Read the model definition and answer for the solid it produces. Units are mm, in the model's axes. A direction names the side the tool comes from. Give positions to 0.01 mm unless a question says otherwise; leave off trailing zeros. Order: outer loops, then holes, each group sorted by start corner. A loop starts at its lowest first (then second) coordinate and runs counter-clockwise, first axis right, second up. Notation, with made-up numbers: M 77.5,26 L 114.5,26 A7 cw 114.5,35 Z; hole C 22,47 d4. An arc over 180 degrees is marked long. One line per item, written item: value. Start each with the question number.
Autodesk Inventor part; units mm, degrees
ref_plane "YZ Plane" through (0, 0, 0) normal (1, 0, 0) x (0, 1, 0)
ref_plane "XZ Plane" through (0, 0, 0) normal (0, 1, 0) x (-1, 0, 0)
ref_plane "XY Plane" through (0, 0, 0) normal (0, 0, 1) x (1, 0, 0)
sketch "Эскиз1" plane through (0, 0, 0) normal (0, 1, 0) x (-1, 0, 0)
  line L0 (150, 150) -> (-150, 150)
  line L1 (-150, 150) -> (-150, -150)
  line L2 (-150, -150) -> (150, -150)
  line L3 (150, -150) -> (150, 150)
  circle A0 centre (0, 0) radius 150
  line L4 (-106, -106) -> (105.4385, -106)
  line L5 (105.4385, -106) -> (105.4385, 106.6899)
  line L6 (105.4385, 106.6899) -> (-106, 106.6899)
  line L7 (-106, 106.6899) -> (-106, -106)
  line L8 (82, 90) -> (-80, 90)
  line L9 (-95, 75) -> (-95, -75)
  line L10 (-80, -90) -> (82, -90)
  line L11 (95, -77) -> (95, 77)
  arc A1 (95, 77) -> (82, 90) centre (82, 77) ccw
  arc A2 (82, -90) -> (95, -77) centre (82, -77) ccw
  line L12 (72, 84.5) -> (12, 84.5)
  line L13 (12, 69.5) -> (72, 69.5)
  line L14 (-80, 90) -> (-82, 90)
  line L15 (-95, 77) -> (-95, 75)
  arc A3 (-82, 90) -> (-95, 77) centre (-82, 77) ccw
  line L16 (-80, -90) -> (-82, -90)
  line L17 (-95, -77) -> (-95, -75)
  arc A4 (-95, -77) -> (-82, -90) centre (-82, -77) ccw
  line L18 (76.9408, 68) -> (82, 68)
  line L19 (82, 68) -> (-82, 68)
  line L20 (-82, 86) -> (82, 86)
  line L21 (82, -68) -> (-82, -68)
  line L22 (-82, -68) -> (-82, -86)
  line L23 (-82, -86) -> (82, -86)
  line L24 (-82, 68) -> (-72, 68)
  line L25 (-72, 86) -> (-82, 86)
  line L26 (-82, 86) -> (-82, 68)
  line L27 (-82, -86) -> (-72, -86)
  line L28 (-72, -68) -> (-82, -68)
  line L29 (-82, -68) -> (-82, -86)
  line L30 (82, -86) -> (72, -86)
  line L31 (72, -68) -> (82, -68)
  line L32 (82, -68) -> (82, -86)
  line L33 (72, 68) -> (82, 68)
  line L34 (82, 68) -> (82, 86)
  line L35 (82, 86) -> (72, 86)
  line L36 (42, 68) -> (54.5, 68)
  line L37 (42, 8) -> (17, 8)
  line L38 (29.5, 8) -> (29.5, 68)
  line L39 (29.5, 68) -> (54.5, 68)
  line L40 (54.5, 68) -> (54.5, 8)
  line L41 (42, -8) -> (17, -8)
  line L42 (29.5, -8) -> (29.5, -68)
  line L43 (29.5, -68) -> (54.5, -68)
  line L44 (54.5, -68) -> (54.5, -8)
  line L45 (-42, 68) -> (-29.5, 68)
  line L46 (-54.5, 8) -> (-54.5, 68)
  line L47 (-54.5, 68) -> (-29.5, 68)
  line L48 (-29.5, 68) -> (-29.5, 8)
  line L49 (-54.5, -8) -> (-54.5, -68)
  line L50 (-54.5, -68) -> (-29.5, -68)
  line L51 (-29.5, -68) -> (-29.5, -8)
  line L52 (75.5, -84.5) -> (8.5, -84.5)
  line L53 (8.5, -84.5) -> (8.5, -69.5)
  line L54 (8.5, -69.5) -> (75.5, -69.5)
  line L55 (75.5, -69.5) -> (75.5, -84.5)
  line L56 (0, -86) -> (0, -44.6693) construction
  line L57 (-75.5, -84.5) -> (-8.5, -84.5)
  line L58 (-8.5, -84.5) -> (-8.5, -69.5)
  line L59 (-8.5, -69.5) -> (-75.5, -69.5)
  line L60 (-75.5, -69.5) -> (-75.5, -84.5)
  line L61 (75.5, 84.5) -> (8.5, 84.5)
  line L62 (8.5, 84.5) -> (8.5, 69.5)
  line L63 (8.5, 69.5) -> (75.5, 69.5)
  line L64 (75.5, 69.5) -> (75.5, 84.5)
  line L65 (-8.5, 84.5) -> (-8.5, 69.5)
  line L66 (-8.5, 69.5) -> (-75.5, 69.5)
  line L67 (-75.5, 69.5) -> (-75.5, 84.5)
  line L68 (-75.5, 84.5) -> (-8.5, 84.5)
  line L69 (54.5, 8) -> (29.5, 8)
  line L70 (17, 8) -> (17, -8)
  line L71 (29.5, -8) -> (54.5, -8)
  line L72 (42, -8) -> (42, 8)
  line L73 (-54.5, 8) -> (-54.5, -8)
  line L74 (-29.5, -8) -> (-29.5, 8)
  line L75 (20, -40) -> (-20, -40)
  line L76 (-20, -40) -> (-20, 40)
  line L77 (-20, 40) -> (20, 40)
  line L78 (20, 40) -> (20, -40)
  line L79 (20, 25) -> (20, 40)
  line L80 (20, 30) -> (20, 40)
  line L81 (-10, -10) -> (10, -10)
  line L82 (10, -10) -> (10, 10)
  line L83 (10, 10) -> (-10, 10)
  line L84 (-10, 10) -> (-10, -10)
  point P0 (-95, -90)
  point P1 (-95, 90)
  point P2 (95, -90)
  point P3 (-12, -77)
  point P4 (12, -77)
  point P5 (12, 77)
  point P6 (72, 77)
  point P7 (42, 8)
  point P8 (42, -8)
  point P9 (-42, -69.5)
  point P10 (42, -8)
  point P11 (-9, 0)
  point P12 (42, 0)
  point P13 (29.5, 0)
  point P14 (-42, -69.5)
  point P15 (42, -69.5)
  dimension "d2" = 300
  dimension "d3" = 300
  dimension "d8" = 190
  dimension "d9" = 180
  dimension "d10" = 13
  dimension "d11" = 13
  dimension "d31" = 13
  dimension "d32" = 13
  dimension "d41" = 15
  dimension "d42" = 24
  dimension "d47" = 25
  dimension "d51" = 25
  dimension "d52" = 16
  dimension "d112" = 67
  dimension "d123" = 40
  dimension "d124" = 80
  dimension "d147" = 20
  dimension "d148" = 20
  dimension "d156" = 84
extrude "Выдавливание1" add sketch "Эскиз1" along normal blind 4 contours A1 L11 A2 L10 L16 A4 L17 L9 L15 A3 L14 L8 | L40 L69 L37 L38 L19 | L38 L37 L78 L77 L76 L75 L41 L42 L21 L51 L74 L48 L19 | L72 L41 L78 L37 | L48 L74 L51 L21 L49 L73 L46 L19 | L71 L44 L21 L42 L41 | L78 L41 L70 L37 | L37 L70 L41 L78 L75 L76 L77 | L84 L83 L82 L81
sketch "Эскиз2" plane through (0, 0, 0) normal (0, -1, 0) x (1, 0, 0)
  line L0 (-82, -68) -> (-82, -86)
  line L1 (-95, -77) -> (-95, 77)
  line L2 (-95, -68) -> (-95, -56.3368)
  line L3 (-95, -45) -> (-95, -68) construction
  line L4 (-95, -68) -> (-80, -68) construction
  line L5 (-95, -63) -> (-95, -68)
  line L6 (-95, -50) -> (-95, -45)
  circle A0 centre (-80, -63) radius 1.5
  circle A1 centre (-80, -50) radius 1.5
  line L7 (95, 77) -> (95, -77)
  line L8 (95, -68) -> (95, -45)
  line L9 (-95, -45) -> (-95, -68)
  line L10 (82, -90) -> (-82, -90)
  circle A2 centre (80, -63) radius 1.5
  circle A3 centre (80, -50) radius 1.5
  line L11 (-95, -68) -> (-95, -63)
  line L12 (95, -63) -> (95, -68)
  line L13 (95, -45) -> (95, -50)
  line L14 (-95, -50) -> (-95, -45)
  circle A4 centre (0, -50) radius 1.5
  circle A5 centre (0, -63) radius 1.5
  line L15 (-95, 0) -> (95, 0)
  circle A6 centre (-80, 63) radius 1.5
  circle A7 centre (-80, 50) radius 1.5
  circle A8 centre (80, 63) radius 1.5
  circle A9 centre (80, 50) radius 1.5
  circle A10 centre (0, 50) radius 1.5
  circle A11 centre (0, 63) radius 1.5
  line L16 (-95, -68) -> (95, -68)
  line L17 (95, -68) -> (95, -45)
  line L18 (95, -45) -> (-95, -45)
  line L19 (-95, -45) -> (-95, -68)
  line L20 (-82, 68) -> (-95, 68)
  line L21 (-95, 68) -> (95, 68)
  line L22 (95, 68) -> (95, 45)
  line L23 (95, 45) -> (-95, 45)
  line L24 (-95, 45) -> (-95, 68)
  point P0 (0, 0)
  dimension "d64" = 23
extrude "Выдавливание2" cut sketch "Эскиз2" against normal blind 4 contours A0 | A1 | A2 | A3 | A4 | A5 | A6 | A7 | A8 | A9 | A10 | A11
sketch "Эскиз3" plane through (0, 0, 0) normal (0, -1, 0) x (1, 0, 0)
  line L0 (-95, -77) -> (-95, 77)
  line L1 (-95, 10) -> (-95, 0)
  circle A0 centre (-73, 0) radius 1.5
  circle A1 centre (-60, -13) radius 1.5
  circle A2 centre (-60, 13) radius 1.5
  line L2 (-70, -10) -> (-80, -10)
  line L3 (-60, -10) -> (-80, -10)
  line L4 (-50, -10) -> (-68, -10)
  line L5 (-70, -8) -> (-70, 8)
  line L6 (-68, 10) -> (-50, 10)
  line L7 (-50, 10) -> (-50, -10)
  arc A3 (-70, -8) -> (-68, -10) centre (-68, -8) ccw
  arc A4 (-68, 10) -> (-70, 8) centre (-68, 8) ccw
  line L8 (0, 0) -> (-42, 0)
  line L9 (-42, 0) -> (-42, 8)
  line L10 (-42, 8) -> (0, 8)
  line L11 (0, 8) -> (0, 0)
  point P0 (-70, -13)
  point P1 (-78, -10)
  point P2 (-70, 0)
  point P3 (-60, 0)
  dimension "d79" = 3
  dimension "d87" = 2
  dimension "d149" = 42
extrude "Выдавливание3" cut sketch "Эскиз3" against normal blind 4 contours A0 | A1 | A2
extrude "Выдавливание4" cut sketch "Эскиз3" against normal blind 4 contours L3 A3 L5 A4 L6 L7 L4
sketch "Эскиз4" plane through (0, 0, 0) normal (0, -1, 0) x (1, 0, 0)
  circle A0 centre (-80, 63) radius 1.5
  circle A1 centre (-78, 57.5) radius 1.5
  circle A2 centre (0, 63) radius 1.5
  circle A3 centre (-2.2, 57.5) radius 1.5
  line L0 (-47.745, 0) -> (17.0058, 0) construction
  circle A4 centre (-78, -57.5) radius 1.5
  circle A5 centre (-2.2, -57.5) radius 1.5
  point P0 (0, 0)
  dimension "d92" = 3
  dimension "d95" = 3
extrude "Выдавливание5" cut sketch "Эскиз4" against normal blind 4 contours A1 | A3 | A4 | A5
sketch "Эскиз5" plane through (0, 0, 0) normal (0, -1, 0) x (1, 0, 0)
  line L0 (82, -68) -> (-82, -68)
  line L1 (-82, -86) -> (82, -86)
  line L2 (-90.0897, 0) -> (-46.8311, 0) construction
  line L3 (0, -13.4429) -> (0, 16.6684) construction
  circle A0 centre (-87, -8.1) radius 1.5
  line L4 (-82, 68) -> (82, 68) construction
  line L5 (0, 68) -> (-4.5, 68) construction
  line L6 (-4.5, 63) -> (0, 63) construction
  line L7 (0, 63) -> (0, 68) construction
  line L8 (-17.2785, 0) -> (16.6341, 0) construction
  circle A1 centre (-8.1, 63) radius 1.5
  circle A2 centre (-87, 8.1) radius 1.5
  circle A3 centre (87, -8.1) radius 1.5
  circle A4 centre (87, 8.1) radius 1.5
  circle A5 centre (8.1, 63) radius 1.5
  circle A6 centre (-8.1, -63) radius 1.5
  circle A7 centre (8.1, -63) radius 1.5
  point P0 (0, 0)
  point P1 (-87, 0)
  dimension "d115" = 3
extrude "Выдавливание6" cut sketch "Эскиз5" against normal blind 4 contours A0
extrude "Выдавливание7" cut sketch "Эскиз5" against normal blind 4 contours A1
extrude "Выдавливание8" cut sketch "Эскиз1" along normal blind 4 contours L72 L41 L78 L37 | L78 L41 L70 L37
extrude "Выдавливание9" cut sketch "Эскиз1" along normal blind 4 contours L84 L83 L82 L81
sketch "Эскиз6" plane through (0, 4, 0) normal (0, 1, 0) x (1, 0, 0)
  line L0 (15, -37.5) -> (75, -37.5)
  line L1 (75, -37.5) -> (75, 37.5)
  line L2 (75, 37.5) -> (15, 37.5)
  line L3 (15, 37.5) -> (15, -37.5)
  line L4 (15, -37.5) -> (25, -37.5)
  line L5 (45, -37.5) -> (45, 37.5) construction
  circle A0 centre (25, 0) radius 1.5
  circle A1 centre (65, 0) radius 1.5
  point P0 (0, 0)
  dimension "d139" = 60
  dimension "d140" = 75
  dimension "d141" = 10
  dimension "d142" = 3
extrude "Выдавливание10" cut sketch "Эскиз6" against normal blind 4 contours A0 | A1
extrude "Выдавливание11" cut sketch "Эскиз5" against normal blind 10 contours A2
extrude "Выдавливание12" cut sketch "Эскиз5" against normal blind 10 contours A3 | A4 | A5 | A6 | A7
properties part number "основа"
Q1. Find section A-A, the plane x = 57. Give the vertices of the cut face in (y, z), then the cut area to 3 significant figures.
Q2. Find section B-B, the plane y = 1.6. State how many separate pieces and enclosed holes the cut face has, then the cut area to 3 significant figures.
Q3. Each of these flat-tipped pins is pushed along its axis until it touches: pin 1 (4 mm diameter, centred on x = 8.1, z = 63, fed in from -Y); pin 2 (2.5 mm diameter, centred on x = 65, z = 0, fed in from -Y); pin 3 (2 mm diameter, centred on y = 2, z = 81.5, fed in from +X). Where does it stop, or does it pass through?
Q4. Consider probe 1 along Z at (x, y) = (-73, 2.4); probe 2 along Z at (x, y) = (-58, 2.3); probe 3 along Z at (x, y) = (-8.1, 2.9). Determine where each line is inside the solid, lowest interval first.
Q5. A tool of negligible diameter and unlimited length cuts with its end or side. For faces 1 (the flat face through (1, 2, -90)), 2 (the flat face through (82, 2, -77)), from which of +Z, -Z, +X, -X, +Y, -Y can it reach the whole face along a straight path? Write none if from no direction.
Q6. Determine the mould class of faces 3 (the cylindrical face through (91.293, 1.972, 86.091)), 4 (the flat face through (-82, 2, 77)), 5 (the cylindrical face through (-91.091, 1.972, 86.293)) for opening direction X: released by +X, released by -X, zero draft, split by the parting line, or undercut.
Evaluation:
1. outline: M 0,-90 L 4,-90 L 4,-86 L 0,-86 Z; M 0,-68 L 4,-68 L 4,68 L 0,68 Z; M 0,86 L 4,86 L 4,90 L 0,90 Z
1. area: 576 mm2
2. separate pieces: 1
2. enclosed holes: 34
2. area: 26,700 mm2
3. pin 1: y = 0
3. pin 2: through
3. pin 3: x = 94.52
4. probe 1: -90 to -86, -68 to -1.5, 1.5 to 68, 86 to 90
4. probe 2: -90 to -86, -68 to -10, 10 to 68, 86 to 90
4. probe 3: -90 to -86, -68 to -64.5, -61.5 to -10, 10 to 61.5, 64.5 to 68, 86 to 90
5. face 1: -Z, +X, -X, +Y, -Y
5. face 2: +Y, -Y
6. face 3: released by +X
6. face 4: undercut
6. face 5: released by -X
